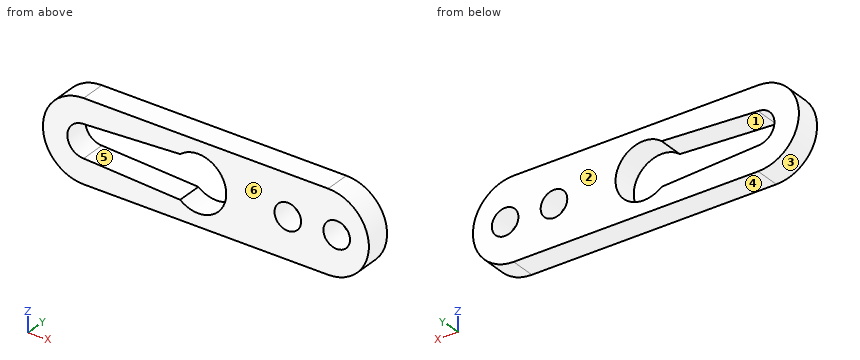
from build123d import *

# Parameters (mm, degrees)
BOSS_EXTRUDE1_DEPTH      = 3
BOSS_EXTRUDE1_DEPTH_BACK = 0.1
F_4_CLEARANCE_HOLE1_D    = 3.2639


with BuildPart() as part:
    # Sketch1 → Boss-Extrude1 (new, two sides: drawn at the far end of the back side and taken through both)
    with BuildSketch(Plane(origin=(0, 0, 0), x_dir=(1, 0, 0), z_dir=(0, 1, 0)).offset(-BOSS_EXTRUDE1_DEPTH_BACK)):
        with BuildLine():
            Line((-15, 5), (15, 5))
            ThreePointArc((15, 5), (20, 0), (15, -5))
            Line((15, -5), (-15, -5))
            ThreePointArc((-15, -5), (-20, 0), (-15, 5))
        make_face()
        with BuildLine():
            Line((-15, 2), (-3.159072307, 2.649999913))
            ThreePointArc((-3.159072307, 2.649999913), (2.5, 0), (-3.159072307, -2.649999913))
            Line((-3.159072307, -2.649999913), (-15, -2))
            ThreePointArc((-15, -2), (-17, 0), (-15, 2))
        make_face(mode=Mode.SUBTRACT)
    extrude(amount=BOSS_EXTRUDE1_DEPTH + BOSS_EXTRUDE1_DEPTH_BACK)

    # #4 Clearance Hole1 (through all)
    with Locations(Plane(origin=(0, 3, 0), x_dir=(1, 0, 0), z_dir=(0, 1, 0))):
        with Locations((10.05, 0), (16.05, 0)):
            Hole(F_4_CLEARANCE_HOLE1_D / 2)


solid = part.part
Check sheet for the modelled part. Datum: model origin and axes. Units: mm. Face numbers are marked on the shaded views. A direction names the side the tool comes from. Give positions to 0.01 mm unless a question says otherwise; leave off trailing zeros. Loops run counter-clockwise (first coordinate to the right, second up) from the corner with the lowest first, then second, coordinate; pieces in that order, holes last. Notation, with made-up numbers: M -34.75,-39.5 L -7.75,-39.5 A22 cw -7.75,-32.5 Z; hole C 15.5,-34.5 d9. An arc over 180 degrees is marked long. Use a Markdown table: item, result. Add a question column.
Q1. Sectioned sample at D-D, the plane x = 10.05. Record the cut outline in (y, z).
Q2. Mould release check, pull along Z, two halves, no side actions. Record for the marked faces 3, 4, 5 and 6: pulls with the +Z half, pulls with the -Z half, needs draft (parallel to the pull), parting line crosses it, or undercut.
Q3. Scan lines: line 1 along Z through (x, y) = (-2.5, 0.95); line 2 along Z through (x, y) = (-10.5, 0.5); line 3 along X through (y, z) = (1.85, -1.75). Record each from-to range of solid material in increasing order. Write a range as [from, to].
Q4. Sectioned sample at C-C, the plane y = 1.7. Record the cut outline in (x, z), then the cut area to 3 significant figures.
Q5. Tool access check on the marked faces 1 and 2. Record the directions out of +Z, -Z, +X, -X, +Y, -Y that give a thin tool (end or side, any length) a straight path to the whole face; none if there is none.
Q6. Sectioned sample at B-B, the plane z = 0. Record the cut outline in (x, y).
Q7. Sectioned sample at A-A, the plane x = -0.95. Record the cut outline in (y, z), then the cut area to 3 significant figures.
Verdict:
| question | item | result |
|---|---|---|
| 1 | outline | M -0.1,-5 L 3,-5 L 3,-1.63 L -0.1,-1.63 Z; M -0.1,1.63 L 3,1.63 L 3,5 L -0.1,5 Z |
| 2 | face 3 | parting line crosses it |
| 2 | face 4 | pulls with the -Z half |
| 2 | face 5 | undercut |
| 2 | face 6 | needs draft |
| 3 | line 1 | [-5, -3.08], [3.08, 5] |
| 3 | line 2 | [-5, -2.25], [2.25, 5] |
| 3 | line 3 | [-19.68, -15.97], [2.02, 19.68] |
| 4 | outline | M -15,-5 L 15,-5 A5 ccw 15,5 L -15,5 A5 ccw Z; hole M -15,-2 L -3.16,-2.65 A3.45 ccw long -3.16,2.65 L -15,2 A2 ccw Z; hole C 10.05,0 d3.26; hole C 16.05,0 d3.26 |
| 4 | area | 268 mm^2 |
| 5 | face 1 | +Y, -Y |
| 5 | face 2 | +Z, -Z, +X, -X, +Y |
| 6 | outline | M -20,-0.1 L -17,-0.1 L -17,3 L -20,3 Z; M 2.5,-0.1 L 8.42,-0.1 L 8.42,3 L 2.5,3 Z; M 11.68,-0.1 L 14.42,-0.1 L 14.42,3 L 11.68,3 Z; M 17.68,-0.1 L 20,-0.1 L 20,3 L 17.68,3 Z |
| 7 | outline | M -0.1,-5 L 3,-5 L 3,-3.45 L -0.1,-3.45 Z; M -0.1,3.45 L 3,3.45 L 3,5 L -0.1,5 Z |
| 7 | area | 9.61 mm^2 |
